Autodesk Inventor part; units mm, degrees
ref_plane "YZ Plane" through (0, 0, 0) normal (1, 0, 0) x (0, 1, 0)
ref_plane "XZ Plane" through (0, 0, 0) normal (0, 1, 0) x (-1, 0, 0)
ref_plane "XY Plane" through (0, 0, 0) normal (0, 0, 1) x (1, 0, 0)
sketch "Sketch2" plane through (0, 0, 0) normal (0, 1, 0) x (-1, 0, 0)
  line L0 (7.9621, 7.1123) -> (-1992.0379, 7.1123)
  line L1 (-1992.0379, 7.1123) -> (-1992.0379, -1992.8877)
  line L2 (-1992.0379, -1992.8877) -> (7.9621, -1992.8877)
  line L3 (7.9621, -1992.8877) -> (7.9621, 7.1123)
  point P0 (0, 0)
  dimension "d0" = 2000
  dimension "d1" = 2000
extrude "Extrusion1" add sketch "Sketch2" along normal blind 320
sketch "Sketch5" plane through (0, 320, 0) normal (0, 1, 0) x (1, 0, 0)
  line L0 (12.0379, 12.8877) -> (1972.0379, 12.8877)
  line L1 (1972.0379, 12.8877) -> (1972.0379, 1972.8877)
  line L2 (1972.0379, 1972.8877) -> (12.0379, 1972.8877)
  line L3 (12.0379, 1972.8877) -> (12.0379, 12.8877)
  line L4 (-7.9621, -7.1123) -> (1992.0379, -7.1123)
  line L5 (1992.0379, -7.1123) -> (1992.0379, 1992.8877)
  dimension "d7" = 1960
  dimension "d8" = 20
  dimension "d9" = 1960
  dimension "d10" = 20
extrude "Extrusion2" cut sketch "Sketch5" against normal blind 300
sketch "Sketch6" plane through (0, 20, 0) normal (0, 1, 0) x (1, 0, 0)
  circle A0 centre (1692.0379, 1692.8877) radius 50
  circle A1 centre (1692.0379, 1542.8877) radius 50
  line L0 (1992.0379, 1992.8877) -> (-7.9621, 1992.8877)
  line L1 (1992.0379, -7.1123) -> (1992.0379, 1992.8877)
  point P0 (0, 0)
  dimension "d13" = 100
  dimension "d14" = 100
  dimension "d15" = 300
  dimension "d16" = 300
  dimension "d17" = 300
  dimension "d18" = 150
extrude "Extrusion3" cut sketch "Sketch6" against normal blind 300
sketch "Sketch7" plane through (0, 0, 0) normal (0, -1, 0) x (1, 0, 0)
  line L0 (1992.0379, 7.1123) -> (1792.0379, 7.1123)
  line L1 (1792.0379, 7.1123) -> (1792.0379, -192.8877)
  line L2 (1792.0379, -192.8877) -> (1992.0379, -192.8877)
  line L3 (1992.0379, -192.8877) -> (1992.0379, 7.1123)
  line L4 (-7.9621, 7.1123) -> (1992.0379, 7.1123)
  line L5 (-7.9621, 7.1123) -> (192.0379, 7.1123)
  line L6 (192.0379, 7.1123) -> (192.0379, -192.8877)
  line L7 (192.0379, -192.8877) -> (-7.9621, -192.8877)
  line L8 (-7.9621, -192.8877) -> (-7.9621, 7.1123)
  line L9 (1792.0379, -1992.8877) -> (1792.0379, -1792.8877)
  line L10 (1792.0379, -1792.8877) -> (1992.0379, -1792.8877)
  line L11 (1992.0379, -1792.8877) -> (1992.0379, -1992.8877)
  line L12 (-7.9621, -1992.8877) -> (192.0379, -1992.8877)
  line L13 (192.0379, -1992.8877) -> (192.0379, -1792.8877)
  line L14 (192.0379, -1792.8877) -> (-7.9621, -1792.8877)
  line L15 (-7.9621, -1792.8877) -> (-7.9621, -1992.8877)
  point P0 (0, 0)
  point P1 (0, -1985.7753)
  dimension "d23" = 200
  dimension "d24" = 200
extrude "Extrusion4" add sketch "Sketch7" along normal blind 500
sketch "Sketch8" plane through (0, 0, 0) normal (0, -1, 0) x (1, 0, 0)
  line L0 (1992.0379, -1992.8877) -> (-7.9621, -1992.8877)
  line L1 (1992.0379, -1992.8877) -> (1792.0379, -1992.8877)
  line L2 (1792.0379, -1992.8877) -> (1792.0379, -1792.8877)
  line L3 (1792.0379, -1792.8877) -> (1992.0379, -1792.8877)
  line L4 (1992.0379, -1792.8877) -> (1992.0379, -1992.8877)
  point P0 (0, 0)
  dimension "d27" = 200
  dimension "d28" = 200
extrude "Extrusion5" add sketch "Sketch8" along normal blind 500
properties part number "grow bed"
Here's how the part is built. I have some questions about the finished solid (model axes, mm). A direction names the side the tool comes from. Round coordinates to 2 decimals unless told otherwise and drop trailing zeros. Write each loop counter-clockwise with the first axis right and the second up, starting at its lowest first coordinate (ties: lowest second). Pieces come first, ordered by that corner, then holes. Notation, with made-up numbers: (7.25, 18.5) -> (54.25, 18.5) arc R25 ccw to (54.25, 47.5) -> close; hole circle Ø3 at (12, -31). An arc over 180 degrees is marked (long way). One line per item, written item: value.
1) If I drill on line 1 (X direction, y = 200, z = -822.5); line 2 (Z direction, x = 1109.5, y = 277); line 3 (Z direction, x = 184.5, y = -379.5), over which ranges is the centre line in solid material (lowest first)? Write a range as [from, to].
Filled sheet:
line 1: x = [-7.96, 12.04], [1972.04, 1992.04]
line 2: z = [-1992.89, -1972.89], [-12.89, 7.11]
line 3: z = [-1992.89, -1792.89], [-192.89, 7.11]
2) I'm going to push a flat-ended pin straight in: pin 1 Ø4 at (x, z) = (537, -628.5) entering from +Y. Where does the tip first touch, or does it pass through?
Filled sheet:
pin 1: stops at y = 20
3) Suppose I cut it at A-A on y = -249. List the corners of the cut face in (x, z) for me, plus the area to 3 significant figures.
Filled sheet:
outline: (-7.96, -1992.89) -> (192.04, -1992.89) -> (192.04, -1792.89) -> (-7.96, -1792.89) -> close; (-7.96, -192.89) -> (192.04, -192.89) -> (192.04, 7.11) -> (-7.96, 7.11) -> close; (1792.04, -1992.89) -> (1992.04, -1992.89) -> (1992.04, -1792.89) -> (1792.04, -1792.89) -> close; (1792.04, -192.89) -> (1992.04, -192.89) -> (1992.04, 7.11) -> (1792.04, 7.11) -> close
area: 160,000 mm2
4) For faces 1 (the face through (1891, -246, -1792.888)), 2 (the face through (192.038, -246, -91)), 3 (the face through (978, 172, -12.888)), which set-ups out of +Z, -Z, +X, -X, +Y, -Y let a thin tool reach every point of the face, with its end or its side?
Filled sheet:
face 1: +X, -X, -Y
face 2: +Z, -Z, -Y
face 3: +Y
5) Suppose I cut it at D-D on x = 567.5. List the corners of the cut face in (y, z) for me.
Filled sheet:
outline: (0, -1992.89) -> (320, -1992.89) -> (320, -1972.89) -> (20, -1972.89) -> (20, -12.89) -> (320, -12.89) -> (320, 7.11) -> (0, 7.11) -> close
6) Suppose I cut it at C-C on y = 74.5. List the corners of the cut face in (x, z) for me, plus the area to 3 significant figures.
Filled sheet:
outline: (-7.96, -1992.89) -> (1992.04, -1992.89) -> (1992.04, 7.11) -> (-7.96, 7.11) -> close; hole (12.04, -1972.89) -> (1972.04, -1972.89) -> (1972.04, -12.89) -> (12.04, -12.89) -> close
area: 158,000 mm2
7) Suppose I cut it at B-B on z = -991. List the corners of the cut face in (x, y) for me.
Filled sheet:
outline: (-7.96, 0) -> (1992.04, 0) -> (1992.04, 320) -> (1972.04, 320) -> (1972.04, 20) -> (12.04, 20) -> (12.04, 320) -> (-7.96, 320) -> close
